Read the model definition and answer for the solid it produces. Units are mm, in the model's axes. A direction names the side the tool comes from. Coordinates: 2 decimals unless noted, no trailing zeros. Write each loop counter-clockwise with the first axis right and the second up, starting at its lowest first coordinate (ties: lowest second). Pieces come first, ordered by that corner, then holes. Notation, with made-up numbers: (-28, 15) -> (-12, 15) arc R15 ccw to (-12, 38) -> close; hole circle Ø2 at (75, 6). An arc over 180 degrees is marked (long way). One line per item, written item: value. Start each with the question number.
from build123d import *

# Parameters (mm, degrees)
SKETCH1_R           = 30
BOSS_EXTRUDE2_DEPTH = 10
SKETCH3_W           = 220
SKETCH3_H           = 80
BOSS_EXTRUDE3_DEPTH = 10
SKETCH4_R           = 40
BOSS_EXTRUDE4_DEPTH = 30


with BuildPart() as part:
    # Sketch1 → Boss-Extrude2 (new body)
    with BuildSketch(Plane.XY):
        with BuildLine():
            Line((0, -50), (-220, -50))
            ThreePointArc((-220, -50), (-270, 0), (-220, 50))
            Line((-220, 50), (0, 50))
            ThreePointArc((0, 50), (50, 0), (0, -50))
        make_face()
        Circle(SKETCH1_R, mode=Mode.SUBTRACT)
    boss_extrude2 = extrude(amount=BOSS_EXTRUDE2_DEPTH)

    # Sketch3 → Boss-Extrude3 (add)
    with BuildSketch(Plane.XZ.offset(50)):
        with Locations((-110, -40)):
            Rectangle(SKETCH3_W, SKETCH3_H)
    boss_extrude3 = extrude(amount=-BOSS_EXTRUDE3_DEPTH)

    # Sketch4 → Boss-Extrude4 (add)
    with BuildSketch(Plane.XY):
        with Locations((-220, 0)):
            Circle(SKETCH4_R)
    boss_extrude4 = extrude(amount=BOSS_EXTRUDE4_DEPTH)

    # Mirror1: Boss-Extrude2, Boss-Extrude3, Boss-Extrude4 across plane
    add(boss_extrude2.mirror(Plane(origin=(0, 0, -35), x_dir=(1, 0, 0), z_dir=(0, 0, -1))))
    add(boss_extrude3.mirror(Plane(origin=(0, 0, -35), x_dir=(1, 0, 0), z_dir=(0, 0, -1))))
    add(boss_extrude4.mirror(Plane(origin=(0, 0, -35), x_dir=(1, 0, 0), z_dir=(0, 0, -1))))

    # Mirror2: Boss-Extrude3 across plane
    add(boss_extrude3.mirror(Plane.ZX))


solid = part.part
1. A tool of negligible diameter and unlimited length cuts with its end or side. For faces 1 (the face through (-259.96, 1.76, 19.86)), 2 (the face through (-112, -40, -35)), 3 (the face through (-220, -45, -35)), from which of +Z, -Z, +X, -X, +Y, -Y can it reach the whole face along a straight path? Write none if from no direction.
2. A cutting plane is placed at B-B on x = -44. Give the vertices of the cut face in (y, z), then the cut area to 3 significant figures.
3. A cutting plane is placed at A-A on z = -60. Give the vertices of the cut face in (x, y).
4. A cutting plane is placed at C-C on y = -24. Give the vertices of the cut face in (x, z), then the cut area to 3 significant figures.
5. Given pin 1 (1.5 mm diameter, centred on x = -26.5, y = -8, fed in from -Z); pin 2 (11 mm diameter, centred on y = -46.5, z = -22, fed in from +X); pin 3 (10 mm diameter, centred on y = -13, z = 5.5, fed in from +X); pin 4 (5 mm diameter, centred on y = -47.5, z = -28.5, fed in from -X), each flat-ended and moving along its own axis, determine where each tip first touches the part or whether it passes through.
6. For a pull along Z with two mould halves and no side action, classify faces 4 (the face through (-112, -50, -34)), 5 (the face through (-108, 1, 10)), 6 (the face through (-108, 1, 0)) as +Z half, -Z half, draft (parallel to the pull), parting line (faces both ways), or undercut.
7. A cutting plane is placed at D-D on x = -4.5. Give the vertices of the cut face in (y, z), then the cut area to 3 significant figures.
8. Find the intervals of material crossed by probe 1 along Z at (x, y) = (-69, 39); probe 2 along Y at (x, z) = (-126, -56); probe 3 along Z at (x, y) = (-238.5, -21), in increasing order. Write a range as from..to.
Derived:
1. face 1: +Z
1. face 2: +X, -X
1. face 3: -X, +Y, -Y
2. outline: (-50, -80) -> (50, -80) -> (50, 10) -> (-50, 10) -> close; hole (-40, -70) -> (40, -70) -> (40, 0) -> (-40, 0) -> close
2. area: 3,400 mm2
3. outline: (-220, -50) -> (0, -50) -> (0, -40) -> (-220, -40) -> close; (-220, 40) -> (0, 40) -> (0, 50) -> (-220, 50) -> close
4. outline: (-263.86, -80) -> (-252, -80) -> (-252, -100) -> (-188, -100) -> (-188, -80) -> (-18, -80) -> (-18, -70) -> (-263.86, -70) -> close; (-263.86, 0) -> (-18, 0) -> (-18, 10) -> (-188, 10) -> (-188, 30) -> (-252, 30) -> (-252, 10) -> (-263.86, 10) -> close; (18, -80) -> (43.86, -80) -> (43.86, -70) -> (18, -70) -> close; (18, 0) -> (43.86, 0) -> (43.86, 10) -> (18, 10) -> close
4. area: 7,990 mm2
5. pin 1: passes through
5. pin 2: stops at x = 0
5. pin 3: stops at x = 49.36
5. pin 4: stops at x = -220
6. face 4: draft
6. face 5: +Z half
6. face 6: undercut
7. outline: (-50, -80) -> (-29.66, -80) -> (-29.66, -70) -> (-40, -70) -> (-40, 0) -> (-29.66, 0) -> (-29.66, 10) -> (-50, 10) -> close; (29.66, -80) -> (50, -80) -> (50, 10) -> (29.66, 10) -> (29.66, 0) -> (40, 0) -> (40, -70) -> (29.66, -70) -> close
7. area: 2,210 mm2
8. probe 1: z = -80..-70, 0..10
8. probe 2: y = -50..-40, 40..50
8. probe 3: z = -100..-70, 0..30
